CAD build for the part. Positions are in the model's coordinates, mm. Face numbers are marked on the shaded views. A direction names the side the tool comes from. Coordinates: 2 decimals unless noted, no trailing zeros. Order: outer loops, then holes, each group sorted by start corner. A loop starts at its lowest first (then second) coordinate and runs counter-clockwise, first axis right, second up. Notation, with made-up numbers: M 82.25,-9 L 107.25,-9 A17 cw 107.25,-1 Z; hole C -8.75,82 d4. An arc over 180 degrees is marked long. Write item = value, one per line. Start each with the question number.
```python
from build123d import *

# Parameters (mm, degrees)
SKETCH1_W           = 90
SKETCH1_H           = 141
BOSS_EXTRUDE1_DEPTH = 2
SKETCH2_W           = 20
SKETCH2_H           = 5
SKETCH2_W_2         = 10
BOSS_EXTRUDE2_DEPTH = 2
SKETCH3_W           = 10
SKETCH3_H           = 2
SKETCH3_W_2         = 20
BOSS_EXTRUDE3_DEPTH = 2
BOSS_EXTRUDE4_DEPTH = 10
FILLET1_R           = 1
FILLET2_R           = 0.5
FILLET3_R           = 0.5
SKETCH5_W           = 25.5
SKETCH5_H           = 47.5
BOSS_EXTRUDE5_DEPTH = 11
FILLET4_R           = 2.5


with BuildPart() as part:
    # Sketch1 → Boss-Extrude1 (new body)
    with BuildSketch(Plane(origin=(0, 0, 0), x_dir=(1, 0, 0), z_dir=(0, 1, 0))):
        Rectangle(SKETCH1_W, SKETCH1_H)
    extrude(amount=BOSS_EXTRUDE1_DEPTH)

    # Sketch2 → Boss-Extrude2 (add)
    with BuildSketch(Plane.XZ):
        with Locations((0, 68)):
            Rectangle(SKETCH2_W, SKETCH2_H)
        with Locations((-38, 68)):
            Rectangle(SKETCH2_W_2, SKETCH2_H)
        with Locations((38, 68)):
            Rectangle(SKETCH2_W_2, SKETCH2_H)
    extrude(amount=BOSS_EXTRUDE2_DEPTH)

    # Sketch3 → Boss-Extrude3 (add)
    with BuildSketch(Plane.XY.offset(70.5)):
        with Locations((-38, -1)):
            Rectangle(SKETCH3_W, SKETCH3_H)
        with Locations((0, -1)):
            Rectangle(SKETCH3_W_2, SKETCH3_H)
        with Locations((38, -1)):
            Rectangle(SKETCH3_W, SKETCH3_H)
    extrude(amount=BOSS_EXTRUDE3_DEPTH)

    # Sketch4 → Boss-Extrude4 (add, symmetric)
    with BuildSketch(Plane.ZY):
        with BuildLine():
            Line((-75.13857422, -1.949748096), (-73.987443964, -8.159637236))
            ThreePointArc((-73.987443964, -8.159637236), (-73, -9.00026478), (-72.012556036, -8.159637236))
            Line((-72.012556036, -8.159637236), (-70.5, 0))
            Line((-70.5, 0), (-70.5, 2))
            Line((-70.5, 2), (-71.146294998, 2))
            Line((-71.146294998, 2), (-72.817734573, -7.016750635))
            ThreePointArc((-72.817734573, -7.016750635), (-73, -7), (-73.182265427, -7.016750635))
            Line((-73.182265427, -7.016750635), (-74.853705002, 2))
            Line((-74.853705002, 2), (-75.5, 2))
            Line((-75.5, 2), (-77.5, 2))
            Line((-77.5, 2), (-77.5, 1))
            Line((-77.5, 1), (-75.6853705, 1))
            Line((-75.6853705, 1), (-75.503105074, 0.016750635))
            ThreePointArc((-75.503105074, 0.016750635), (-76.304089012, -1.148764157), (-75.13857422, -1.949748096))
        make_face()
    extrude(amount=BOSS_EXTRUDE4_DEPTH, both=True)

    # Fillet1
    fillet1_edges = [part.edges().sort_by_distance(p)[0] for p in [
        (0, 0, -70.5),
    ]]
    fillet(fillet1_edges, radius=FILLET1_R)

    # Fillet2
    fillet2_edges = [part.edges().sort_by_distance(p)[0] for p in [
        (0, 2, -71.146294998),
        (0, 2, -74.853705002),
    ]]
    fillet(fillet2_edges, radius=FILLET2_R)

    # Fillet3
    fillet3_edges = [part.edges().sort_by_distance(p)[0] for p in [
        (0, 1, -75.6853705),
    ]]
    fillet(fillet3_edges, radius=FILLET3_R)

    # Sketch5 → Boss-Extrude5 (add)
    with BuildSketch(Plane.XZ):
        Polygon((33, 50.5), (33, 60.5), (28, 60.5), (28, 50.5), (2.5, 50.5), (2.5, 60.5), (-2.5, 60.5), (-2.5, 50.5), (-28, 50.5), (-28, 60.5), (-33, 60.5), (-33, 50.5), (-40, 50.5), (-40, 48.5), (-33, 48.5), (-33, 1), (-40, 1), (-40, -1), (-33, -1), (-33, -48.5), (-40, -48.5), (-40, -50.5), (-33, -50.5), (-33, -60.5), (-28, -60.5), (-28, -50.5), (-2.5, -50.5), (-2.5, -60.5), (2.5, -60.5), (2.5, -50.5), (28, -50.5), (28, -60.5), (33, -60.5), (33, -50.5), (40, -50.5), (40, -48.5), (33, -48.5), (33, -1), (40, -1), (40, 1), (33, 1), (33, 48.5), (40, 48.5), (40, 50.5), align=None)
        with Locations((-15.25, -24.75)):
            Rectangle(SKETCH5_W, SKETCH5_H, mode=Mode.SUBTRACT)
        with Locations((15.25, -24.75)):
            Rectangle(SKETCH5_W, SKETCH5_H, mode=Mode.SUBTRACT)
        with Locations((-15.25, 24.75)):
            Rectangle(SKETCH5_W, SKETCH5_H, mode=Mode.SUBTRACT)
        with Locations((15.25, 24.75)):
            Rectangle(SKETCH5_W, SKETCH5_H, mode=Mode.SUBTRACT)
    extrude(amount=BOSS_EXTRUDE5_DEPTH)

    # Fillet4
    fillet4_edges = [part.edges().sort_by_distance(p)[0] for p in [
        (-40, -11, 49.5),
        (-40, -11, 0),
        (-40, -11, -49.5),
        (30.5, -11, -60.5),
        (30.5, -11, 60.5),
        (0, -11, 60.5),
        (-30.5, -11, 60.5),
        (-30.5, -11, -60.5),
        (0, -11, -60.5),
        (40, -11, -49.5),
        (40, -11, 0),
        (40, -11, 49.5),
    ]]
    fillet(fillet4_edges, radius=FILLET4_R)


solid = part.part
```
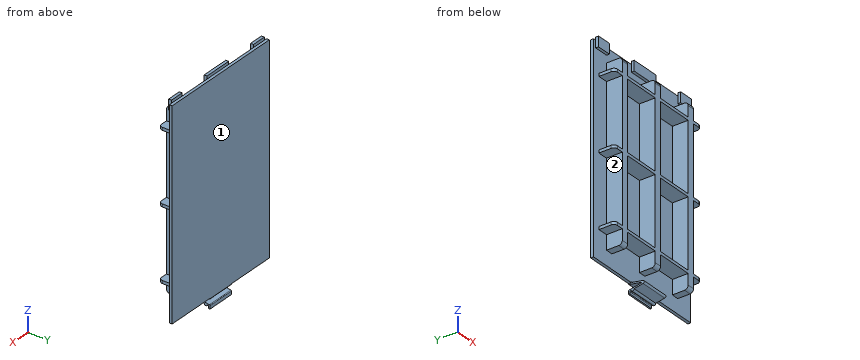
1. Slice it at D-D (x = 36). Write the cut outline in (y, z), plus the area to 3 significant figures.
2. Flat gauge pins, fed straight in: pin 1 (3.5 mm diameter, centred on x = -18.5, y = -5.5, fed in from +Z); pin 2 (1.5 mm diameter, centred on y = -5.5, z = 41.5, fed in from -X); pin 3 (6 mm diameter, centred on x = -1.5, y = -2.5, fed in from -Z). Where does each tip first touch, or does it go through?
3. Slice it at A-A (z = -10). Write the cut outline in (x, y), plus the area to 3 significant figures.
4. 3-axis set-ups, long thin cutter, end or side, ignore diameter. For the marked faces 1 and 2: which of +Z, -Z, +X, -X, +Y, -Y reach the whole face in a straight line?
5. Probe L1, parallel to Z at x = 3.5, y = -8.25; L2, parallel to X at y = -0.5, z = 23; L3, parallel to Z at x = -11, y = -1. List the from-to ranges inside material, lowest first.
6. Slice it at C-C (y = -4). Give the number of separate pieces and of enclosed holes in the cut face, plus the area to 3 significant figures.
Calculated:
q1.outline = M -11,-50.5 L 0,-50.5 L 0,-70.5 L 2,-70.5 L 2,70.5 L 0,70.5 L 0,72.5 L -2,72.5 L -2,65.5 L 0,65.5 L 0,50.5 L -11,50.5 L -11,48.5 L 0,48.5 L 0,1 L -11,1 L -11,-1 L 0,-1 L 0,-48.5 L -11,-48.5 Z
q1.area = 362 mm²
q2.pin_1 = 50.5
q2.pin_2 = -33
q2.pin_3 = -76.32
q3.outline = M -45,0 L -33,0 L -33,-11 L -28,-11 L -28,0 L -2.5,0 L -2.5,-11 L 2.5,-11 L 2.5,0 L 28,0 L 28,-11 L 33,-11 L 33,0 L 45,0 L 45,2 L -45,2 Z
q3.area = 345 mm²
q4.face_1 = +Z, -Z, +X, -X, +Y
q4.face_2 = -X, -Y
q5.L1 = -73.97 to -72.03, -50.5 to -48.5, -1 to 1, 48.5 to 50.5
q5.L2 = -33 to -28, -2.5 to 2.5, 28 to 33
q5.L3 = -50.5 to -48.5, -1 to 1, 48.5 to 50.5
q6.separate_pieces = 3
q6.enclosed_holes = 4
q6.area = 2,250 mm²
